Can you work these out from the model? Positions are in its coordinate system, mm. Face numbers are marked on the shaded views. A direction names the side the tool comes from. Give positions to 0.01 mm unless a question says otherwise; leave off trailing zeros. Loops run counter-clockwise (first coordinate to the right, second up) from the corner with the lowest first, then second, coordinate; pieces in that order, holes last.
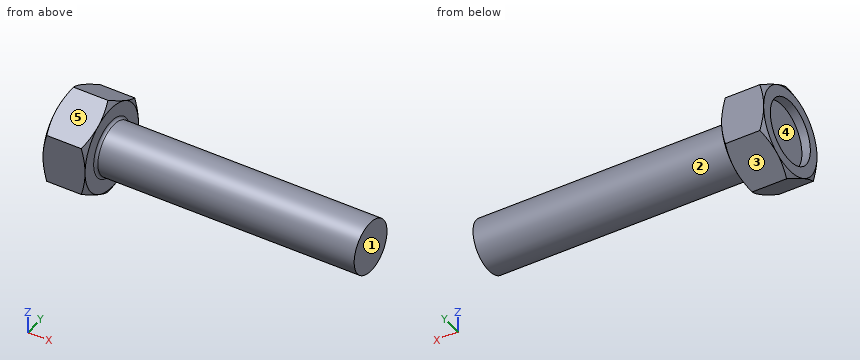
Autodesk Inventor part; units mm, degrees
ref_plane "Work Plane1" through (3, 0, 0) normal (0, 0.5, 0.866) x (1, 0, 0)
ref_plane "YZ Plane" through (0, 0, 0) normal (1, 0, 0) x (0, 1, 0)
ref_plane "XZ Plane" through (0, 0, 0) normal (0, 1, 0) x (-1, 0, 0)
sketch "Sketch1" plane through (0, 0, 0) normal (0, 0, 1) x (1, 0, 0)
  line L0 (0, 4) -> (0, 0)
  line L1 (0, 0) -> (40, 0)
  line L2 (40, 0) -> (40, 4)
  line L3 (40, 4) -> (0, 4)
  line L4 (-8, 0) -> (48, 0)
  line L5 (0, -0.8) -> (0, 4.8)
  dimension "d0" = 8
  dimension "d1" = 40
revolve "Body" add sketch "Sketch1" angle 360 about axis through (0, 0, 0) along (1, 0, 0)
sketch "Sketch2" plane through (0, 0, 0) normal (1, 0, 0) x (0, 1, 0)
  line L0 (0, 7.5056) -> (6.5, 3.7528)
  line L1 (6.5, 3.7528) -> (6.5, -3.7528)
  line L2 (6.5, -3.7528) -> (0, -7.5056)
  line L3 (0, -7.5056) -> (-6.5, -3.7528)
  line L4 (-6.5, -3.7528) -> (-6.5, 3.7528)
  line L5 (-6.5, 3.7528) -> (0, 7.5056)
  line L6 (-9.1, 0) -> (9.1, 0)
  line L7 (0, -10.5078) -> (0, 10.5078)
  point P0 (0, 0)
  point P1 (0, 0)
  dimension "d2" = 13
extrude "Head" add sketch "Sketch2" against normal blind 6.5
sketch "Sketch3" plane through (-6.5, 0, 0) normal (-1, 0, 0) x (0, 1, 0)
  circle A0 centre (0, 0) radius 4.875
  point P0 (0, 0)
  dimension "d12" = 9.75
extrude "Indent1" cut sketch "Sketch3" against normal blind 1.3
sketch "Sketch4" plane through (0, 0, 0) normal (0, 0, 1) x (1, 0, 0)
  line L0 (-6.5, 7.5056) -> (-6.5, 6.5)
  line L1 (-6.5, 6.5) -> (-5.9194, 7.5056)
  line L2 (-5.9194, 7.5056) -> (-6.5, 7.5056)
  line L3 (0, 7.5056) -> (0, 6.5)
  line L4 (0, 6.5) -> (-0.5806, 7.5056)
  line L5 (-0.5806, 7.5056) -> (0, 7.5056)
  line L6 (0, 0) -> (-6.5, 0)
  line L7 (-6.5, 0) -> (-6.5, 6.5)
  line L8 (0, 0) -> (0, 6.5)
  line L9 (-7.8, 0) -> (1.3, 0)
  line L10 (-5.9194, 7.5056) -> (-0.5806, 7.5056) construction
  line L11 (0, -1.5011) -> (0, 9.0067)
  dimension "d6" = 30
  dimension "d7" = 30
  dimension "d16" = 13
  dimension "d17" = 13
  dimension "d18" = 15.0111
revolve "Chamfer1" cut sketch "Sketch4" angle 360 about axis through (-10, 0, 0) along (1, 0, 0)
fillet "Fillet1" radius 0.4 1 edges at (0, -4, 0)
thread "Thread"
ref_plane "Work Plane1" through (3, 0, 0) normal (0, 0.5, 0.866) x (1, 0, 0)
equation "\"d0\" = GD"
equation "\"d1\" = NLG"
equation "\"d2\" = SW"
equation "\"d3\" = KOH"
equation "\"d12\" = 0.75 * SW0"
equation "\"d14\" = 0.2 * KOH"
equation "\"d6\" = ANG1"
equation "\"d7\" = ANG1"
equation "\"d16\" = SW0"
equation "\"d17\" = SW0"
equation "\"d18\" = 1.1547 * SW"
equation "\"d11\" = RR"
equation "\"d8\" = GEL"
equation "\"NLG\" = 40"
equation "\"KOH\" = 6.5"
equation "\"GD\" = NND"
equation "\"GEL\" = 37.5"
equation "\"SW\" = 13"
equation "\"SW0\" = SW"
equation "\"ANG1\" = 30deg"
equation "\"RR\" = 0.4"
equation "\"GUL\" = 0.61345 * PTC"
equation "\"SPD\" = NND - 1.2269 * PTC"
equation "\"GD1\" = THREADDIA - 1.2269 * PTC"
equation "\"THREADDIA\" = 8"
equation "\"SDH\" = 9.2"
equation "\"TOA\" = 30deg"
equation "\"BDM\" = NND"
equation "\"FAWI\" = 45deg"
equation "\"PTC\" = 1.25"
equation "\"NND\" = 8"
equation "\"GAL\" = 0.61345 * PTC"
equation "\"SD\" = 0"
equation "\"SD2\" = SDH"
equation "\"E0\" = 1.155 * SW"
properties part number "AS 1427 - M8 x 40" material "Steel, Mild"
(1) Will these pins go through, and if not, where does the flat tip stop? P1, Ø1.5, axis at x = 6.5, z = -2, coming from the +Y side; P2, Ø2, axis at y = 3, z = 4.5, coming from the +X side; P3, Ø2, axis at x = 13, y = 3.5, coming from the +Z side.
Returned:
P1: stops at y = 3.8
P2: stops at x = 0
P3: stops at z = 3.12
(2) Suppose I cut it at A-A on x = 4.5. List the corners of the cut face in (y, z) for me.
Returned:
outline: circle Ø8 at (0, 0)
(3) Thinking about a two-plate mould opening in Y: for the marked faces 3, 4 and 5, which applies, pulls with the +Y half, pulls with the -Y half, needs draft (parallel to the pull), parting line crosses it, or undercut?
Returned:
face 3: pulls with the +Y half
face 4: undercut
face 5: pulls with the -Y half
(4) Please list where these lines run through material, in increasing order: probe 1 along Y at (x, z) = (-6.1, 0) (3 decimals); probe 2 along X at (y, z) = (-0.5, -3.75); probe 3 along X at (y, z) = (3.25, 4.5).
Returned:
probe 1: y = -6.5 to -4.875, 4.875 to 6.5
probe 2: x = -5.2 to 40
probe 3: x = -6.5 to 0
(5) Which directions (+Z, -Z, +X, -X, +Y, -Y) give clear straight access to the entire face, cutting with the end or side of a thin tool? Please do the marked faces 1 and 2.
Returned:
face 1: +Z, -Z, +X, +Y, -Y
face 2: +X
